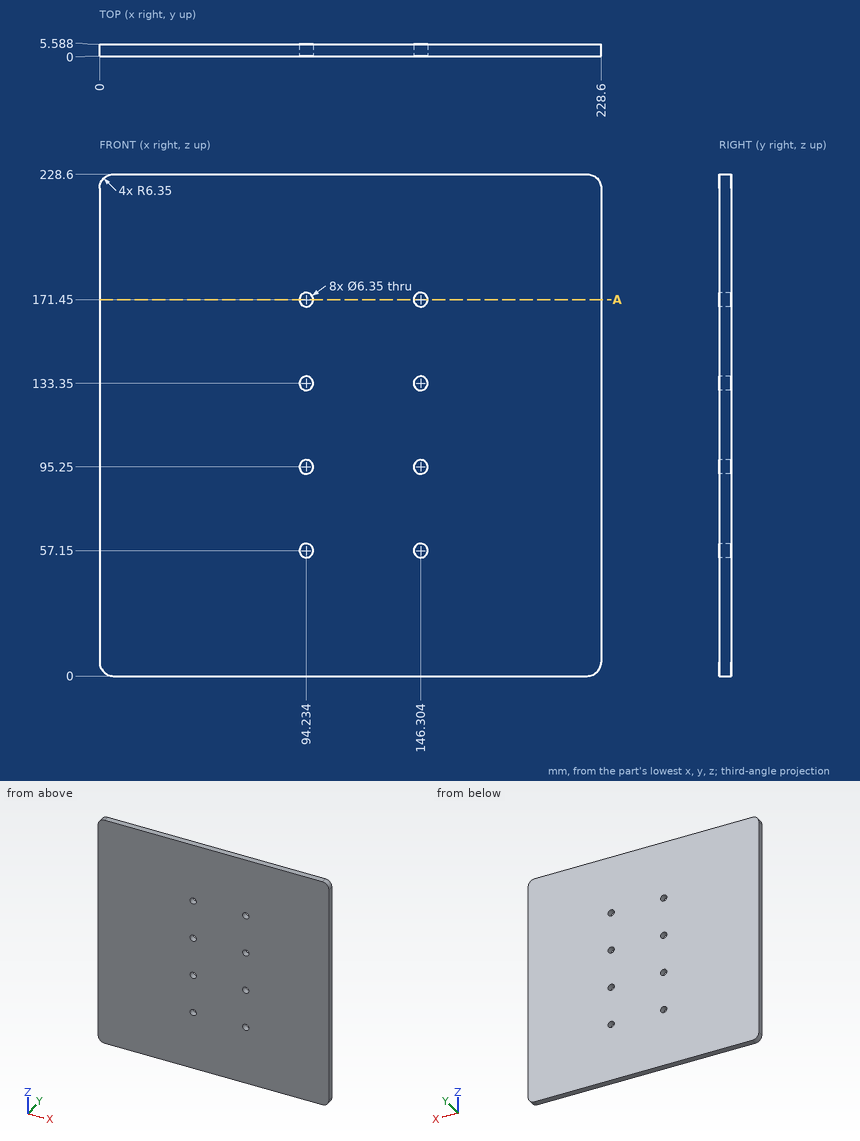
Answer from the drawing. Dimensions are ordinates in mm from the lowest x, y and z of the part. Give positions to 0.01 mm unless a question says otherwise; leave off trailing zeros. Order: outer loops, then holes, each group sorted by start corner. A loop starts at its lowest first (then second) coordinate and runs counter-clockwise, first axis right, second up.
(1) Straight lines are drawn through the part: L1, parallel to X at y = 1.8, z = 57.15; L2, parallel to Z at x = 95, y = 4.95. For each, find the intervals that lie inside material, in ascending order.
(2) Find section A-A (z = 171.45). Give the vertices of the cut face in (x, y), plus the area to 3 significant figures.
(3) Given pin 1 (5 mm diameter, centred on x = 94.234, z = 95.25, fed in from +Y), flat-ended and moving along its own axis, determine where the tip first touches the part or whether it passes through.
Result sheet:
1. L1: x = 0 to 91.06, 97.41 to 143.13, 149.48 to 228.6
1. L2: z = 0 to 54.07, 60.23 to 92.17, 98.33 to 130.27, 136.43 to 168.37, 174.53 to 228.6
2. outline: (0, 0) - (91.06, 0) - (91.06, 5.59) - (0, 5.59) - close; (97.41, 0) - (143.13, 0) - (143.13, 5.59) - (97.41, 5.59) - close; (149.48, 0) - (228.6, 0) - (228.6, 5.59) - (149.48, 5.59) - close
2. area: 1,210 mm2
3. pin 1: passes through
